Build history of the part. All positions in model axes, mm. Face numbers are marked on the shaded views. Round coordinates to 2 decimals unless told otherwise and drop trailing zeros. Write each loop counter-clockwise with the first axis right and the second up, starting at its lowest first coordinate (ties: lowest second). Pieces come first, ordered by that corner, then holes. Notation, with made-up numbers: M 43,88 L 97,88 A14 ccw 97,101 Z; hole C -38,69 d8. An arc over 180 degrees is marked long. Use a Markdown table: item, result.
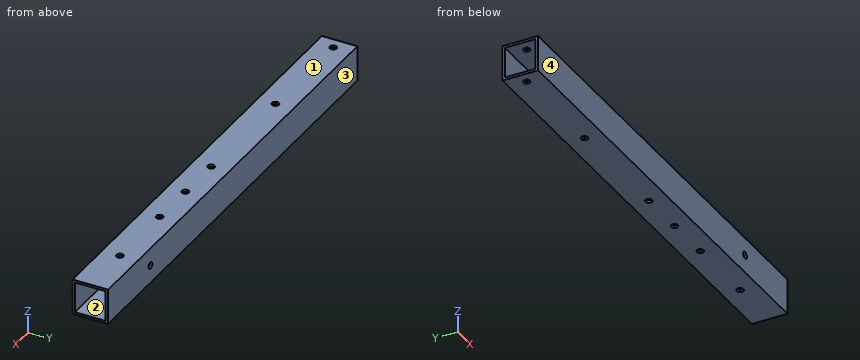
from build123d import *

# Parameters (mm, degrees)
SKETCH_11_W         = 15
SKETCH_11_H         = 15
SKETCH_11_W_2       = 13
SKETCH_11_H_2       = 13
F_15X15X1_1_DEPTH   = 194
SKETCH_12_R         = 1.45
CUT_EXTRUDE_1_DEPTH = 195.723521948
SKETCH_13_R         = 1.45
CUT_EXTRUDE_2_DEPTH = 195.723521948
SKETCH_14_R         = 1.45
CUT_EXTRUDE_3_DEPTH = 195.723521948
SKETCH_15_R         = 1.45
CUT_EXTRUDE_4_DEPTH = 195.723521948


with BuildPart() as part:
    # 草图11 → 铝管 15X15X1(1) (new body)
    with BuildSketch(Plane(origin=(0, 0, 0), x_dir=(0, 0, -1), z_dir=(1, 0, 0))):
        Rectangle(SKETCH_11_W, SKETCH_11_H)
        Rectangle(SKETCH_11_W_2, SKETCH_11_H_2, mode=Mode.SUBTRACT)
    extrude(amount=F_15X15X1_1_DEPTH)

    # 草图12 → 切除-拉伸1 (cut, through all)
    with BuildSketch(Plane(origin=(0, 0, -7.5), x_dir=(-1, 0, 0), z_dir=(0, 0, -1))):
        with Locations((-5, 0)):
            Circle(SKETCH_12_R)
        with Locations((-50, 0)):
            Circle(SKETCH_12_R)
    extrude(amount=-CUT_EXTRUDE_1_DEPTH, mode=Mode.SUBTRACT)

    # 草图13 → 切除-拉伸2 (cut, through all)
    with BuildSketch(Plane(origin=(0, 0, -7.5), x_dir=(-1, 0, 0), z_dir=(0, 0, -1))):
        with Locations((-171, 0)):
            Circle(SKETCH_13_R)
    extrude(amount=-CUT_EXTRUDE_2_DEPTH, mode=Mode.SUBTRACT)

    # 草图14 → 切除-拉伸3 (cut, through all)
    with BuildSketch(Plane(origin=(0, 7.5, 0), x_dir=(1, 0, 0), z_dir=(0, 1, 0))):
        with Locations(Location((161, 0, 0), (0, 0, 270))):
            Circle(SKETCH_14_R)
    extrude(amount=-CUT_EXTRUDE_3_DEPTH, mode=Mode.SUBTRACT)

    # 草图15 → 切除-拉伸4 (cut, through all)
    with BuildSketch(Plane(origin=(0, 0, -7.5), x_dir=(-1, 0, 0), z_dir=(0, 0, -1))):
        with Locations((-120, 0)):
            Circle(SKETCH_15_R)
        with Locations((-140, 0)):
            Circle(SKETCH_15_R)
        with Locations((-100, 0)):
            Circle(SKETCH_15_R)
    extrude(amount=-CUT_EXTRUDE_4_DEPTH, mode=Mode.SUBTRACT)


solid = part.part
Q1. Drop a flat-ended pin along its axis: P1, Ø2.5, axis at x = 100, y = 0, coming from the -Z side. Give the stop position or say it passes through.
Response values:
| item | result |
|---|---|
| P1 | passes through |
Q2. Cut at B-B on y = -4.5. Give the cut face in (x, z), and give its area (3 significant figures).
Response values:
| item | result |
|---|---|
| outline | M 0,-7.5 L 194,-7.5 L 194,-6.5 L 0,-6.5 Z; M 0,6.5 L 194,6.5 L 194,7.5 L 0,7.5 Z |
| area | 388 mm2 |
Q3. Two-plate mould, pull along Y, no slides. Class the marked faces 1, 2, 3 and 4: +Y half, -Y half, draft (parallel to the pull), parting line (faces both ways), or undercut.
Response values:
| item | result |
|---|---|
| face 1 | draft |
| face 2 | undercut |
| face 3 | +Y half |
| face 4 | -Y half |
Q4. Cut at A-A on x = 110.5. Give the cut face in (y, z), and give its area (3 significant figures).
Response values:
| item | result |
|---|---|
| outline | M -7.5,-7.5 L 7.5,-7.5 L 7.5,7.5 L -7.5,7.5 Z; hole M -6.5,-6.5 L 6.5,-6.5 L 6.5,6.5 L -6.5,6.5 Z |
| area | 56.0 mm2 |
Q5. Drill centre lines: L1, parallel to Y at x = 140, z = 6.7; L2, parallel to Y at x = 98.5, z = -4.5. Where is each one in solid material? Low to high.
Response values:
| item | result |
|---|---|
| L1 | y = -7.5 to -1.45, 1.45 to 7.5 |
| L2 | y = -7.5 to -6.5, 6.5 to 7.5 |
